Check sheet for the modelled part. Datum: model origin and axes. Units: mm. Round coordinates to 2 decimals unless told otherwise and drop trailing zeros. Order: outer loops, then holes, each group sorted by start corner. A loop starts at its lowest first (then second) coordinate and runs counter-clockwise, first axis right, second up.
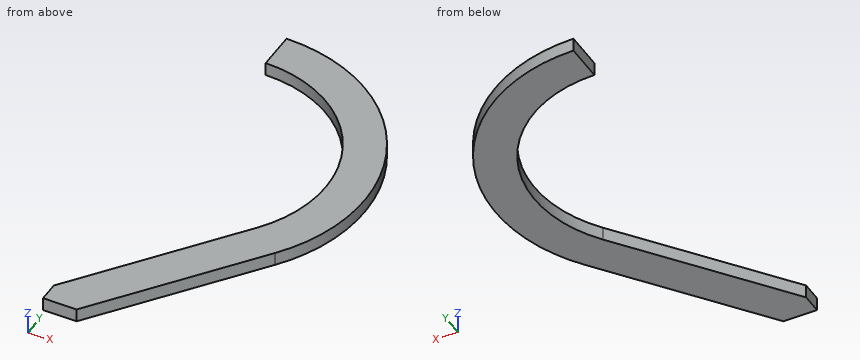
Autodesk Inventor part; units mm, degrees
ref_plane "YZ Plane" through (0, 0, 0) normal (1, 0, 0) x (0, 1, 0)
ref_plane "XZ Plane" through (0, 0, 0) normal (0, 1, 0) x (-1, 0, 0)
ref_plane "XY Plane" through (0, 0, 0) normal (0, 0, 1) x (1, 0, 0)
sketch "Skizze1" plane through (0, 0, 0) normal (0, 0, 1) x (1, 0, 0)
  line L0 (0, 0) -> (5, 0)
  line L1 (5, 0) -> (22.3624, 22.7154)
  arc A0 (22.3624, 22.7154) -> (2.5, 62.8971) centre (2.5, 37.8971) ccw
  line L2 (2.5, 62.8971) -> (2.5, 57.1029)
  arc A1 (17.7589, 26.2341) -> (2.5, 57.1029) centre (2.5, 37.8971) ccw
  line L3 (17.7589, 26.2341) -> (0, 3)
  line L4 (0, 3) -> (0, 0)
  point P0 (2.5, 0)
  point P1 (2.5, 60)
  dimension "d0" = 3
  dimension "d1" = 5
  dimension "d2" = 25
  dimension "d3" = 60
extrude "Extrusion1" add sketch "Skizze1" along normal blind 2
properties part number "LEDholderv_3D-Druck"
1) Sectioned sample at C-C on x = 4. Record the cut outline in (y, z).
2) Gauge pin test, flat ends, axial feed: pin 1 (1 mm diameter, centred on x = 19, z = 0.5, fed in from -Y); pin 2 (1 mm diameter, centred on y = 39, z = 1, fed in from -X); pin 3 (1 mm diameter, centred on y = 59.5, z = 1.5, fed in from -X). Record the tip position at first contact, or that the pin passes through.
3) Sectioned sample at B-B on z = 1.5. Record the cut outline in (x, y), and give its area (3 significant figures).
4) Scan lines: line 1 (Y direction, x = 7.75, z = 0.8); line 2 (Y direction, x = 5.5, z = 0.3); line 3 (Y direction, x = 24.75, z = 1.05). Record each from-to range of solid material in increasing order.
5) Sectioned sample at D-D on y = 53.5. Record the cut outline in (x, z).
6) Sectioned sample at A-A on x = 13.75. Record the cut outline in (y, z), and give its area (3 significant figures).
Values found:
1. outline: (0, 0) - (8.23, 0) - (8.23, 2) - (0, 2) - close; (57.04, 0) - (62.85, 0) - (62.85, 2) - (57.04, 2) - close
2. pin 1: stops at y = 17.66
2. pin 2: stops at x = 21.64
2. pin 3: stops at x = 2.5
3. outline: (0, 0) - (5, 0) - (22.36, 22.72) arc R25 ccw to (2.5, 62.9) - (2.5, 57.1) arc R19.21 cw to (17.76, 26.23) - (0, 3) - close
3. area: 460 mm2
4. line 1: y = 3.6 to 13.14, 56.37 to 62.34
4. line 2: y = 0.65 to 10.2, 56.87 to 62.72
4. line 3: y = 26.5 to 49.3
5. outline: (13.7, 0) - (22.03, 0) - (22.03, 2) - (13.7, 2) - close
6. outline: (11.45, 0) - (20.99, 0) - (20.99, 2) - (11.45, 2) - close; (53.46, 0) - (60.22, 0) - (60.22, 2) - (53.46, 2) - close
6. area: 32.6 mm2
